Part print with two shaded views. Sizes in mm from the minimum x, y, z corner. A direction names the side the tool comes from. Round coordinates to 2 decimals unless told otherwise and drop trailing zeros. Loops run counter-clockwise (first coordinate to the right, second up) from the corner with the lowest first, then second, coordinate; pieces in that order, holes last. Notation, with made-up numbers: M 20,-22 L 56,-22 A27 ccw 56,7 Z; hole C -32.5,70.5 d9. An arc over 180 degrees is marked long. Use a Markdown table: item, result. Add a question column.
Item 1: Wall check: L1, parallel to X at y = 26, z = 40; L2, parallel to Y at x = 8, z = 28.5; L3, parallel to Z at x = 131, y = 15.5. Give the ranges that are in metal, low to high. Write a range as from..to.
Item 2: Saw through at A-A on z = 28. Write the cut outline in (x, y).
Item 3: Saw through at C-C on y = 7. Write the cut outline in (x, z), then the cut area to 3 significant figures.
Item 4: Saw through at D-D on z = 18. Write the cut outline in (x, y), then the cut area to 4 significant figures.
Item 5: Saw through at B-B on y = 16.5. Write the cut outline in (x, z).
Item 6: Pin check, flat tips, straight feed: P1, Ø13, axis at x = 4, z = 30.5, coming from the -Y side; P2, Ø6, axis at x = 6.5, z = 30.5, coming from the +Y side; P3, Ø2.5, axis at x = 7, y = 15.5, coming from the +Z side. Stop position of each tip, or through.
Item 7: Tool access for the marked faces 1, 2 and 3: list every direction of +Z, -Z, +X, -X, +Y, -Y with a clear straight run to the whole face (end or side of a thin tool).
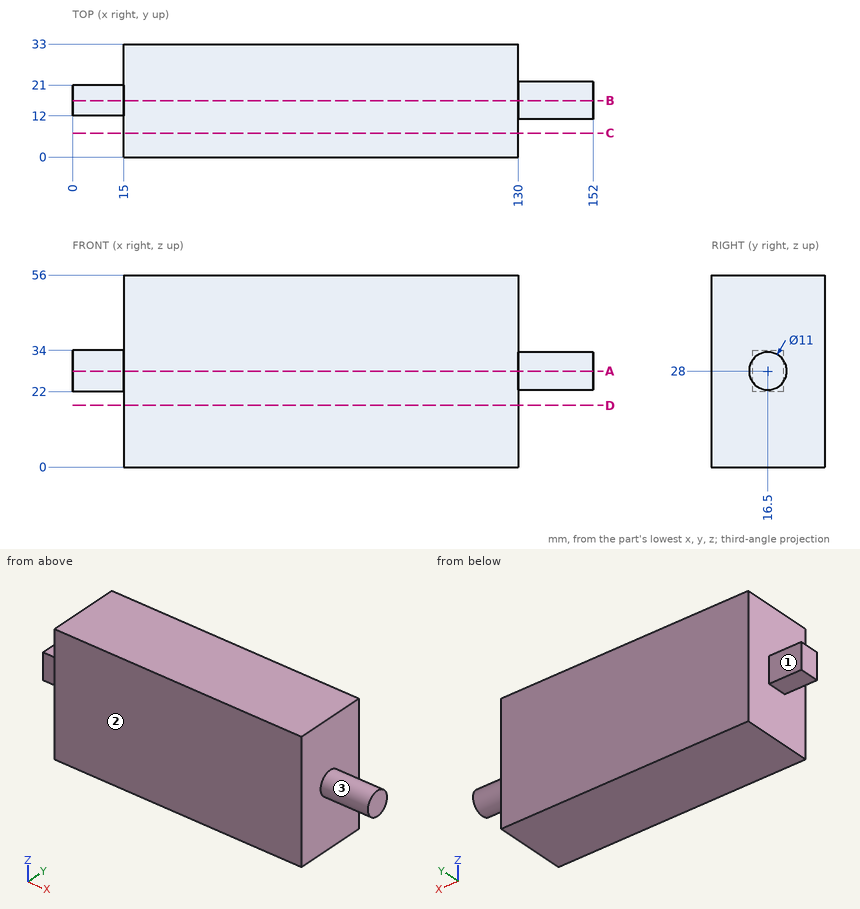
Entries:
| question | item | result |
|---|---|---|
| 1 | L1 | 15..130 |
| 1 | L2 | 12..21 |
| 1 | L3 | 22.59..33.41 |
| 2 | outline | M 0,12 L 15,12 L 15,0 L 130,0 L 130,11 L 152,11 L 152,22 L 130,22 L 130,33 L 15,33 L 15,21 L 0,21 Z |
| 3 | outline | M 15,0 L 130,0 L 130,56 L 15,56 Z |
| 3 | area | 6,440 mm2 |
| 4 | outline | M 15,0 L 130,0 L 130,33 L 15,33 Z |
| 4 | area | 3,795 mm2 |
| 5 | outline | M 0,22 L 15,22 L 15,0 L 130,0 L 130,22.5 L 152,22.5 L 152,33.5 L 130,33.5 L 130,56 L 15,56 L 15,34 L 0,34 Z |
| 6 | P1 | y = 12 |
| 6 | P2 | y = 21 |
| 6 | P3 | z = 34 |
| 7 | face 1 | +Z, -Z, -X, +Y |
| 7 | face 2 | +Z, -Z, +X, -X, -Y |
| 7 | face 3 | +X |
